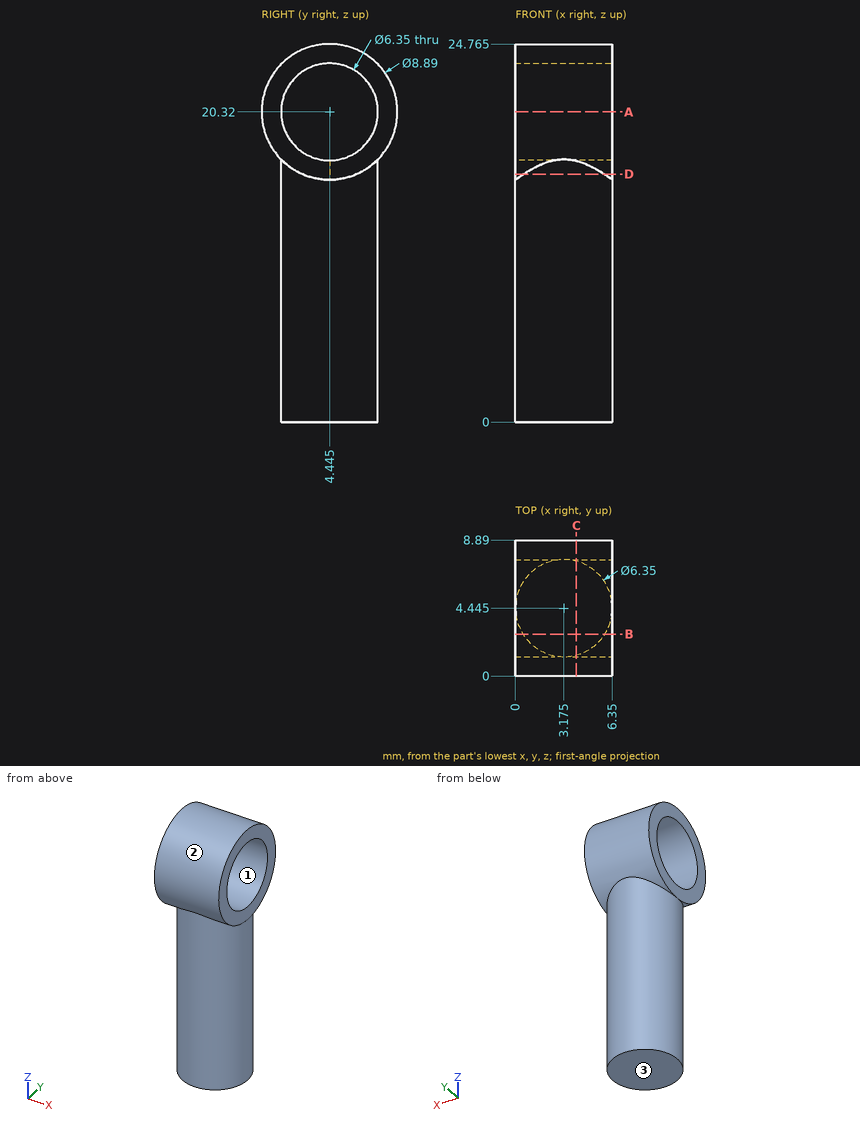
Geometry: see drawing. Coordinates: mm, zero at the bounding-box minimum. Give positions to 0.01 mm unless a question says otherwise; leave off trailing zeros. Order: outer loops, then holes, each group sorted by start corner. A loop starts at its lowest first (then second) coordinate and runs counter-clockwise, first axis right, second up.
Q1. Section B-B on y = 2.75. Output: boundary loops of the cut face in (x, z), and give its area (3 significant figures).
Checked values:
outline: (0, 16.21) - (0.49, 16.21) - (0.49, 0) - (5.86, 0) - (5.86, 16.21) - (6.35, 16.21) - (6.35, 17.64) - (0, 17.64) - close; (0, 23) - (6.35, 23) - (6.35, 24.43) - (0, 24.43) - close
area: 105 mm2
Q2. Contact query for a flat-ended pin moving along its axis: pin 1 Ø3 at (y, z) = (6.5, 7) entering from -X. Output: stop coordinate, or through.
Checked values:
pin 1: stops at x = 0.05
Q3. Section C-C on x = 4. Output: boundary loops of the cut face in (y, z) (3 decimals), and give its area (3 significant figures).
Checked values:
outline: (1.379, 0) - (7.511, 0) - (7.511, 17.102) arc R4.445 ccw (long way) to (1.379, 17.102) - close; hole circle Ø6.35 at (4.445, 20.32)
area: 130 mm2
Q4. Section A-A on z = 20.32. Output: boundary loops of the cut face in (x, y), and give its area (3 significant figures).
Checked values:
outline: (0, 0) - (6.35, 0) - (6.35, 1.27) - (0, 1.27) - close; (0, 7.62) - (6.35, 7.62) - (6.35, 8.89) - (0, 8.89) - close
area: 16.1 mm2
Q5. Ray query, probe 1 along Y at (x, z) = (1.5, 20.32); probe 2 along Y at (x, z) = (1.5, 21); probe 3 along Z at (x, y) = (4, 4.5). Return the intervals inside material, ascending.
Checked values:
probe 1: y = 0 to 1.27, 7.62 to 8.89
probe 2: y = 0.05 to 1.34, 7.55 to 8.84
probe 3: z = 0 to 17.15, 23.49 to 24.76
Q6. Draft query along Y for the marked faces 1, 2 and 3. Return one class per face: +Y half, -Y half, draft (parallel to the pull), parting line (faces both ways), or undercut.
Checked values:
face 1: undercut
face 2: parting line
face 3: draft
Q7. Section D-D on z = 16.25. Output: boundary loops of the cut face in (x, y) (3 decimals).
Checked values:
outline: (0, 2.658) - (0.551, 2.658) arc R3.175 ccw to (5.799, 2.658) - (6.35, 2.658) - (6.35, 6.232) - (5.799, 6.232) arc R3.175 ccw to (0.551, 6.232) - (0, 6.232) - close
